The drawing under review shows one solid part. Ordinate dimensions are in mm from its lowest x, y, z. A direction names the side the tool comes from. Coordinates: 2 decimals unless noted, no trailing zeros. Write each loop counter-clockwise with the first axis right and the second up, starting at its lowest first coordinate (ties: lowest second). Pieces come first, ordered by that corner, then holes.
Q1. Take a section at C-C (y = 80.5). Give the boundary of the cut face in (x, z).
Q2. Machinability: for the marked faces 1, 2, 3, 4 and 5, which of the approach directions +Z, -Z, +X, -X, +Y, -Y give a long, thin tool a straight path to every point of the face, cutting with its end or side? Answer none if there is none.
Q3. Mouldability with a two-part tool opening along X and no side actions: class the marked faces 6, 7, 8 and 9 as pulls with the +X half, pulls with the -X half, needs draft (parallel to the pull), parting line crosses it, or undercut.
Q4. Take a section at B-B (y = 31.5). Give the boundary of the cut face in (x, z), and give its area (3 significant figures).
Q5. Take a section at A-A (x = 17). Give the boundary of the cut face in (y, z), and give its area (3 significant figures).
Q6. For probe 1 along Y at (x, z) = (16, 11.25); probe 2 along Y at (x, z) = (29.5, 1.75); probe 3 along X at (y, z) = (11.5, 5.25), list the stretches that pass through material, from the lowest coordinate up.
Q7. Insertion check: pin 1 (5 mm diameter, centred on x = 27.5, z = 1.5, fed in from +Y); pin 2 (4 mm diameter, centred on x = 36, z = 8, fed in from -Y); pin 3 (6.5 mm diameter, centred on x = 25, y = 14.5, fed in from +Z); pin 4 (15 mm diameter, centred on x = 35, y = 82.5, fed in from -Z). Each pin has a flat end and moves straight along its axis. Give the tip position at first contact, or say it passes through.
Q8. Take a section at D-D (z = 7.5). Give the boundary of the cut face in (x, y), and give its area (3 significant figures).
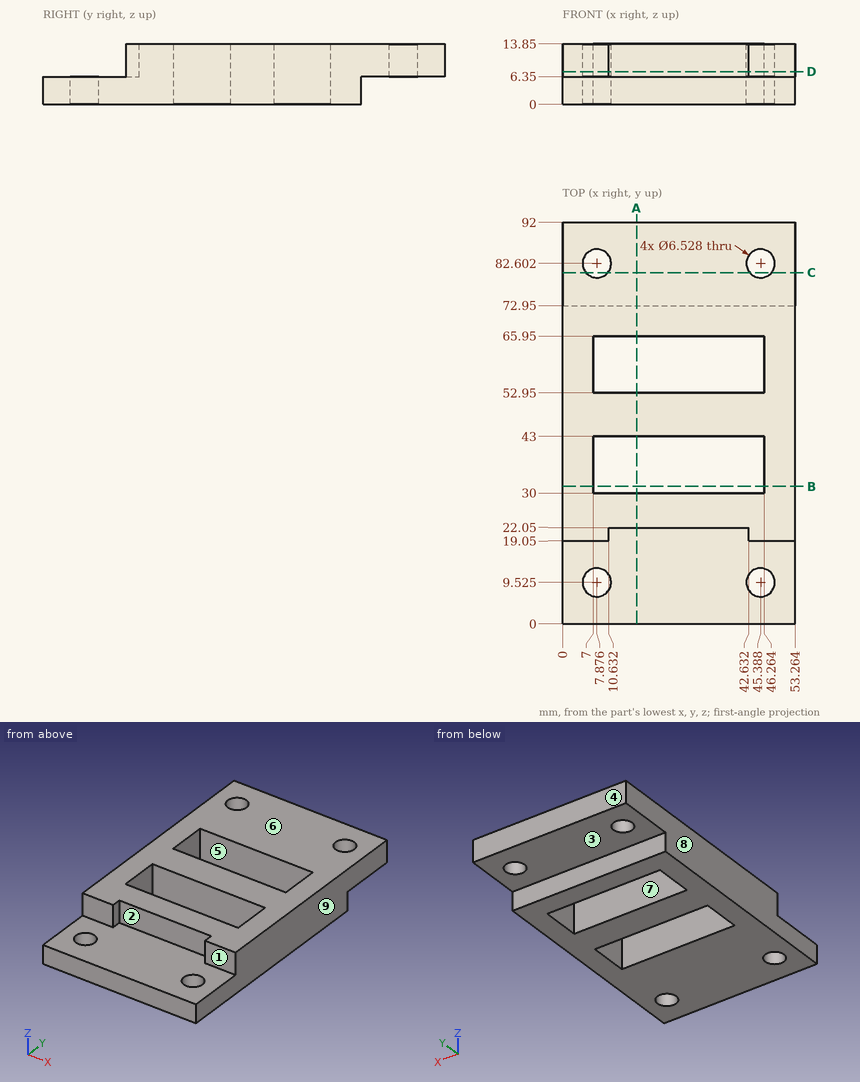
Response:
1. outline: (0, 6.35) - (5.38, 6.35) - (5.38, 13.85) - (0, 13.85) - close; (10.37, 6.35) - (42.89, 6.35) - (42.89, 13.85) - (10.37, 13.85) - close; (47.89, 6.35) - (53.26, 6.35) - (53.26, 13.85) - (47.89, 13.85) - close
2. face 1: +Z, +X, -X, -Y
2. face 2: +Z, -Y
2. face 3: -Z, +X, -X, +Y
2. face 4: +Z, -Z, +X, -X, +Y
2. face 5: +Z, -Z
3. face 6: needs draft
3. face 7: undercut
3. face 8: pulls with the -X half
3. face 9: pulls with the +X half
4. outline: (0, 0) - (7, 0) - (7, 13.85) - (0, 13.85) - close; (46.26, 0) - (53.26, 0) - (53.26, 13.85) - (46.26, 13.85) - close
4. area: 194 mm2
5. outline: (0, 0) - (30, 0) - (30, 13.85) - (22.05, 13.85) - (22.05, 6.35) - (0, 6.35) - close; (43, 0) - (52.95, 0) - (52.95, 13.85) - (43, 13.85) - close; (65.95, 0) - (72.95, 0) - (72.95, 6.35) - (92, 6.35) - (92, 13.85) - (65.95, 13.85) - close
5. area: 628 mm2
6. probe 1: y = 22.05 to 30, 43 to 52.95, 65.95 to 92
6. probe 2: y = 0 to 30, 43 to 52.95, 65.95 to 72.95
6. probe 3: x = 0 to 5.28, 10.47 to 42.79, 47.99 to 53.26
7. pin 1: stops at y = 72.95
7. pin 2: stops at y = 0
7. pin 3: stops at z = 6.35
7. pin 4: stops at z = 6.35
8. outline: (0, 19.05) - (10.63, 19.05) - (10.63, 22.05) - (42.63, 22.05) - (42.63, 19.05) - (53.26, 19.05) - (53.26, 92) - (0, 92) - close; hole circle Ø6.53 at (7.88, 82.6); hole (7, 30) - (46.26, 30) - (46.26, 43) - (7, 43) - close; hole (7, 52.95) - (46.26, 52.95) - (46.26, 65.95) - (7, 65.95) - close; hole circle Ø6.53 at (45.39, 82.6)
8. area: 2,700 mm2
